```python
from build123d import *

# Parameters (mm, degrees)
F0_R      = 8
F1_DEPTH  = 3.7
F2_R      = 6
F3_DEPTH  = 5.8
F4_R      = 8
F5_DEPTH  = 8.7
F6_R      = 12.5
F7_DEPTH  = 32
F8_R      = 2.200771
F9_DEPTH  = 4.8
F10_W     = 16
F10_H     = 16
F11_DEPTH = 12
F13_DEPTH = 5
F14_SIZE  = 3


with BuildPart() as f1:
    # F0 (on Top) → F1 (new body)
    with BuildSketch(Plane.XY):
        Circle(F0_R)
    extrude(amount=F1_DEPTH)

    # F2 (on face) → F3 (join)
    with BuildSketch(Plane(origin=(0, 0, 0), x_dir=(1, 0, 0), z_dir=(0, 0, -1))):
        Circle(F2_R)
    extrude(amount=F3_DEPTH)

    # F4 (on face) → F5 (join)
    with BuildSketch(Plane(origin=(0, 0, -5.8), x_dir=(1, 0, 0), z_dir=(0, 0, -1))):
        Circle(F4_R)
    extrude(amount=F5_DEPTH)

    # F6 (on face) → F7 (join)
    with BuildSketch(Plane(origin=(0, 0, -14.5), x_dir=(1, 0, 0), z_dir=(0, 0, -1))):
        Circle(F6_R)
    extrude(amount=F7_DEPTH)

    # F8 (on face) → F9 (join)
    with BuildSketch(Plane(origin=(0, 0, -46.5), x_dir=(1, 0, 0), z_dir=(0, 0, -1))):
        Circle(F8_R)
    extrude(amount=F9_DEPTH)

    # F10 (on face) → F11 (join)
    with BuildSketch(Plane(origin=(0, 0, -51.3), x_dir=(1, 0, 0), z_dir=(0, 0, -1))):
        with Locations((0, 4)):
            Rectangle(F10_W, F10_H)
    extrude(amount=F11_DEPTH)

    # F12 (on face) → F13 (join)
    with BuildSketch(Plane(origin=(0, 0, -63.3), x_dir=(1, 0, 0), z_dir=(0, 0, -1))):
        Polygon((2, 3.464102), (-2, 3.464102), (-4, 0), (-2, -3.464102), (2, -3.464102), (4, 0), align=None)
    extrude(amount=F13_DEPTH)

    # F14
    f14_edges = [f1.edges().sort_by_distance(p)[0] for p in [
        (0, -3.464102, -68.3),
        (-3, -1.732051, -68.3),
        (-3, 1.732051, -68.3),
        (0, 3.464102, -68.3),
        (3, 1.732051, -68.3),
        (3, -1.732051, -68.3),
    ]]
    chamfer(f14_edges, length=F14_SIZE)


solid = f1.part
```
Input: part model. Units: mm. Frame: model coordinates. A direction names the side the tool comes from. Coordinates: 2 decimals unless noted, no trailing zeros. Write each loop counter-clockwise with the first axis right and the second up, starting at its lowest first coordinate (ties: lowest second). Pieces come first, ordered by that corner, then holes.
1) Section A-A on y = -7. Output: boundary loops of the cut face in (x, z), and give its area (3 significant figures).
2) Section B-B on z = -8.5. Output: boundary loops of the cut face in (x, y).
3) Section C-C on z = -23. Output: boundary loops of the cut face in (x, y), and give its area (3 significant figures).
4) Set-up query: faces 1 (the flat face through (8, -4, -57)), 2 (the cylindrical face through (-0.477, 2.148, -48.866)), 3 (the flat face through (2.986, 1.756, -64.286)), 4 (the flat face through (0, -3.464, -64)). Return all of +Z, -Z, +X, -X, +Y, -Y with unobstructed straight access to the full face (end or side cutting, diameter ignored); none if empty.
5) Section D-D on y = 10.25. Output: boundary loops of the cut face in (x, z).
6) Pin query (flat end, axial travel): pin 1 Ø9.5 at (y, z) = (-1, -59) entering from +X; pin 2 Ø3 at (x, z) = (-9.5, -32) entering from -Y; pin 3 Ø1.6 at (x, z) = (0, -64.5) entering from -Y. Return the tip coordinate at first contact, or that it passes through.
7) Material intervals for line 1 along Z through (x, y) = (-2.75, -5.75); line 2 along Z through (x, y) = (2.5, 5.5); line 3 along Z through (x, y) = (-6.75, -7.5), sorted ascending.
8) Mould query, pull axis Z, two halves, no side actions, for faces 5 (the flat face through (-1.957, -1.162, -66.488)), 6 (the flat face through (-2.986, -1.756, -64.286)), 7 (the flat face through (-2, -6, -5.8)). Classes: pulls with the +Z half, pulls with the -Z half, needs draft (parallel to the pull), parting line crosses it, or undercut.
Check result:
1. outline: (-10.36, -46.5) - (10.36, -46.5) - (10.36, -14.5) - (3.87, -14.5) - (3.87, -5.8) - (-3.87, -5.8) - (-3.87, -14.5) - (-10.36, -14.5) - close; (-8, -63.3) - (8, -63.3) - (8, -51.3) - (-8, -51.3) - close; (-3.87, 0) - (3.87, 0) - (3.87, 3.7) - (-3.87, 3.7) - close
1. area: 951 mm2
2. outline: circle Ø16 at (0, 0)
3. outline: circle Ø25 at (0, 0)
3. area: 491 mm2
4. face 1: -Z, +X, +Y, -Y
4. face 2: none
4. face 3: -Z, +X, +Y
4. face 4: -Z, +X, -X, -Y
5. outline: (-7.15, -46.5) - (7.15, -46.5) - (7.15, -14.5) - (-7.15, -14.5) - close
6. pin 1: stops at x = 8
6. pin 2: stops at y = -9.6
6. pin 3: stops at y = -3.46
7. line 1: z = -63.3 to -51.3, -46.5 to -5.8, 0 to 3.7
7. line 2: z = -46.5 to -5.8, 0 to 3.7
7. line 3: z = -63.3 to -51.3, -46.5 to -14.5
8. face 5: pulls with the -Z half
8. face 6: needs draft
8. face 7: undercut
